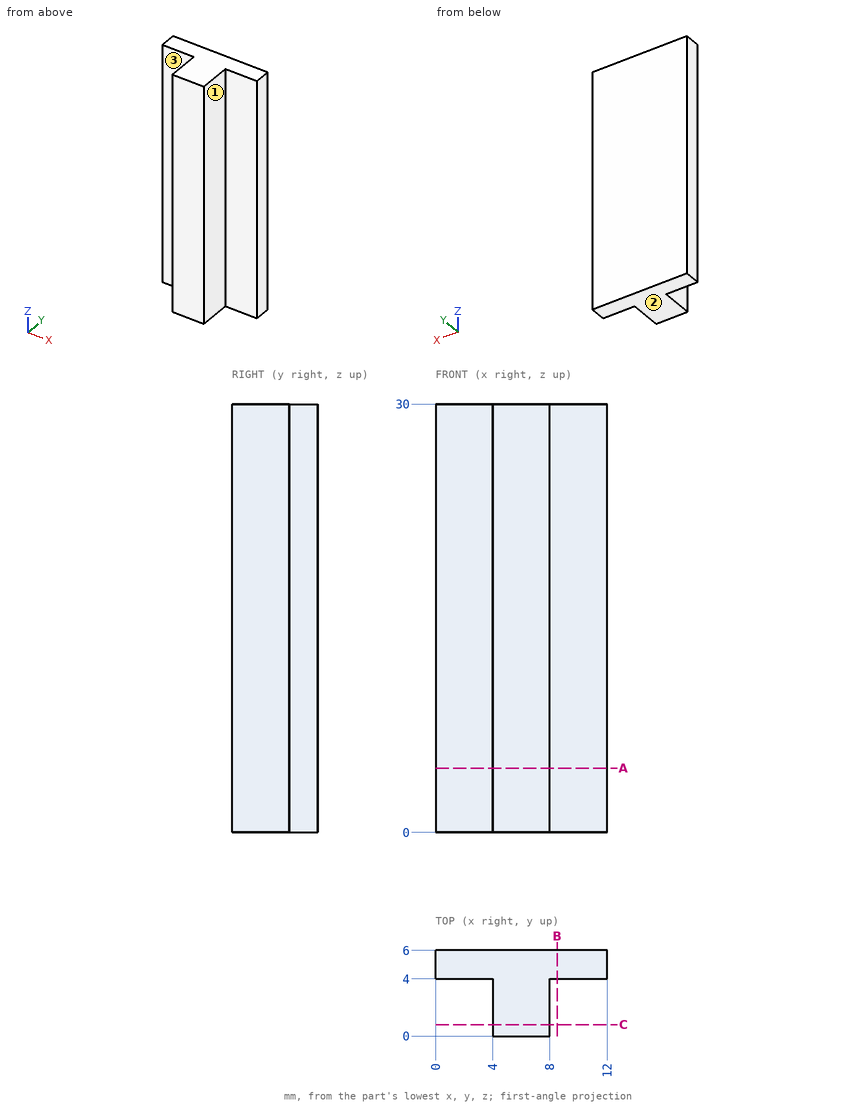
Could you check a few things on this drawing? It's one solid part, dimensions in mm from its lowest x, y, z. A direction names the side the tool comes from. Round coordinates to 2 decimals unless told otherwise and drop trailing zeros. Loops run counter-clockwise (first coordinate to the right, second up) from the corner with the lowest first, then second, coordinate; pieces in that order, holes last. Notation, with made-up numbers: M -9.5,-28 L 38.5,-28 A23 ccw 38.5,-5 Z; hole C -16.5,51 d11. An arc over 180 degrees is marked long. Write each question's results on one line, items separated by ' | '. Start each with the question number.
(1) Will these pins go through, and if not, where does the flat tip stop? P1, Ø1.2, axis at x = 2, z = 20, coming from the -Y side; P2, Ø1.2, axis at y = 2, z = 20, coming from the -X side; P3, Ø1.2, axis at y = 2.5, z = 16.5, coming from the +X side; P4, Ø1.5, axis at x = 1.5, y = 2.5, coming from the +Z side.
(2) I want a section at B-B (x = 8.5). Please give me the cut outline in (y, z), then the cut area to 3 significant figures.
(3) On a 3-axis mill with a long thin cutter (end or side, diameter ignored), from which of +Z, -Z, +X, -X, +Y, -Y can I reach the whole of each face in a straight line? I mean the marked faces 1, 2 and 3. Say none if no direction works.
(4) I want a section at A-A (z = 4.5). Please give me the cut outline in (x, y).
(5) I want a section at C-C (y = 0.8). Please give me the cut outline in (x, z).
(6) If I drill on probe 1 along Y at (x, z) = (10.5, 23.75); probe 2 along X at (y, z) = (0.6, 8), over which ranges is the centre line in solid material (lowest first)? Write a range as from..to.
Solved:
1) P1: stops at y = 4 | P2: stops at x = 4 | P3: stops at x = 8 | P4: passes through
2) outline: M 4,0 L 6,0 L 6,30 L 4,30 Z | area: 60.0 mm²
3) face 1: +Z, -Z, +X, -Y | face 2: -Z, +X, -X, +Y, -Y | face 3: +Z, -Z, -X, -Y
4) outline: M 0,4 L 4,4 L 4,0 L 8,0 L 8,4 L 12,4 L 12,6 L 0,6 Z
5) outline: M 4,0 L 8,0 L 8,30 L 4,30 Z
6) probe 1: y = 4..6 | probe 2: x = 4..8
